Autodesk Inventor part; units mm, degrees
ref_plane "YZ Plane" through (0, 0, 0) normal (1, 0, 0) x (0, 1, 0)
ref_plane "XZ Plane" through (0, 0, 0) normal (0, 1, 0) x (-1, 0, 0)
ref_plane "XY Plane" through (0, 0, 0) normal (0, 0, 1) x (1, 0, 0)
sketch "Sketch1" plane through (0, 0, 0) normal (0, 0, 1) x (1, 0, 0)
  line L0 (-75, -42.5) -> (75, -42.5)
  line L1 (75, -42.5) -> (75, 42.5)
  line L2 (75, 42.5) -> (-75, 42.5)
  line L3 (-75, 42.5) -> (-75, -42.5)
  line L4 (-75, -42.5) -> (75, 42.5) construction
  line L5 (75, -42.5) -> (-75, 42.5) construction
  circle A0 centre (55, -22.5) radius 10
  circle A1 centre (55, 22.5) radius 10
  line L6 (0, 0) -> (75, 0) construction
  circle A2 centre (55, 0) radius 10
  dimension "d0" = 150
  dimension "d1" = 85
  dimension "d23" = 20
  dimension "d25" = 20
  dimension "d26" = 20
extrude "Plate1" add sketch "Sketch1" along normal blind 8 contours L3 L2 L1 L0 | A0 | A1
fillet "Corner Round1" radius 5 4 edges at (75, -42.5, 4) (-75, -42.5, 4) (-75, 42.5, 4) (75, 42.5, 4)
sketch "Sketch5" plane through (0, 0, 8) normal (0, 0, 1) x (1, 0, 0)
  line L0 (70, -42.5) -> (-70, -42.5)
  line L1 (-75, -37.5) -> (-75, 37.5)
  line L2 (-70, 42.5) -> (70, 42.5)
  circle A0 centre (-32.5, 0) radius 42.5
  circle A1 centre (-32.5, 0) radius 5
  point P0 (0, 0)
  dimension "d27" = 10
extrude "Extrusion2" cut sketch "Sketch5" against normal blind 1 contours A1
equation "\"d26\" = d25"
equation "\"d2\" = Thickness"
equation "\"BendReliefWidth\" = Thickness"
equation "\"BendReliefDepth\" = 0.5 * Thickness"
equation "\"CornerReliefSize\" = 4 * Thickness"
equation "\"MinimumRemnant\" = 2 * Thickness"
equation "\"TransitionRadius\" = BendRadius"
equation "\"JacobiRadiusSize\" = BendRadius"
equation "\"GapSize\" = Thickness"
properties part number "PNS-783 leg floor plate" material "Steel"
Could you check a few things on this model? Use its own coordinates, in mm. A direction names the side the tool comes from. Round coordinates to 2 decimals unless told otherwise and drop trailing zeros. Write each loop counter-clockwise with the first axis right and the second up, starting at its lowest first coordinate (ties: lowest second). Pieces come first, ordered by that corner, then holes. Notation, with made-up numbers: (69, -26.75) - (121, -26.75) arc R12 cw to (121, -18.75) - close; hole circle Ø9 at (0.25, -4.5). An arc over 180 degrees is marked (long way). Use a Markdown table: item, result.
Q1. I want a section at B-B (x = 55). List the corners of the cut face in (y, z) for me, plus the area to 3 significant figures.
Output values:
| item | result |
|---|---|
| outline | (-42.5, 0) - (-10, 0) - (-10, 8) - (-42.5, 8) - close; (10, 0) - (42.5, 0) - (42.5, 8) - (10, 8) - close |
| area | 520 mm2 |
Q2. I want a section at C-C (z = 4.75). List the corners of the cut face in (x, y) for me, plus the area to 3 significant figures.
Output values:
| item | result |
|---|---|
| outline | (-75, -37.5) arc R5 ccw to (-70, -42.5) - (70, -42.5) arc R5 ccw to (75, -37.5) - (75, 37.5) arc R5 ccw to (70, 42.5) - (-70, 42.5) arc R5 ccw to (-75, 37.5) - close; hole circle Ø20 at (55, 0) |
| area | 12,400 mm2 |
Q3. Thinking about a two-plate mould opening in X: for faces 1 (the flat face through (-1, 1, 0)), 2 (the cylindrical face through (73.57, 41, 4.06)), 3 (the flat face through (-33, 0, 7)), which applies, released by +X, released by -X, zero draft, split by the parting line, or undercut?
Output values:
| item | result |
|---|---|
| face 1 | zero draft |
| face 2 | released by +X |
| face 3 | undercut |
Q4. For pin 1 (3 mm diameter, centred on x = -35, y = -0.5, fed in from +Z), with a flat end and sliding along its axis, tell me the tip position at first contact or that it passes through.
Output values:
| item | result |
|---|---|
| pin 1 | z = 7 |
Q5. Please list where these lines run through material, in increasing order: L1, parallel to X at y = 3.5, z = 4.5; L2, parallel to X at y = -6.5, z = 0.5.
Output values:
| item | result |
|---|---|
| L1 | -75 to 45.63, 64.37 to 75 |
| L2 | -75 to 47.4, 62.6 to 75 |
Q6. I want a section at A-A (y = 0). List the corners of the cut face in (x, z) for me, plus the area to 3 significant figures.
Output values:
| item | result |
|---|---|
| outline | (-75, 0) - (45, 0) - (45, 8) - (-27.5, 8) - (-27.5, 7) - (-37.5, 7) - (-37.5, 8) - (-75, 8) - close; (65, 0) - (75, 0) - (75, 8) - (65, 8) - close |
| area | 1,030 mm2 |
Q7. For faces 4 (the flat face through (1, 42.5, 4)), 5 (the cylindrical face through (-37.495, 0.22, 7.507)), which set-ups out of +Z, -Z, +X, -X, +Y, -Y let a thin tool reach every point of the face, with its end or its side?
Output values:
| item | result |
|---|---|
| face 4 | +Z, -Z, +X, -X, +Y |
| face 5 | +Z |
